```python
from build123d import *

# Parameters (mm, degrees)
F0_W     = 1.376042
F0_H     = 15
F1_DEPTH = 19
F2_R     = 5
F3_R     = 4.06
F4_DEPTH = 17
F5_R     = 4.15
F5_R_2   = 2.15
F6_DEPTH = 3


with BuildPart() as f1:
    # F0 (on Top) → F1 (new body)
    with BuildSketch(Plane.XY):
        with BuildLine():
            ThreePointArc((-27.724563, 11.37891), (-27.434191, 12.156994), (-27.831811, 12.886122))
            ThreePointArc((-27.831811, 12.886122), (-30.832093, 14.457622), (-34.175314, 15))
            Line((-34.175314, 15), (-34.175314, 12.15))
            ThreePointArc((-34.175314, 12.15), (-31.784278, 11.77065), (-29.628073, 10.669856))
            ThreePointArc((-29.628073, 10.669856), (-28.961501, 10.481293), (-28.332327, 10.771145))
            Line((-28.332327, 10.771145), (-27.724563, 11.37891))
        make_face()
        with BuildLine():
            Line((-34.175314, 12.15), (-34.175314, 15))
            ThreePointArc((-34.175314, 15), (-43.081071, 10.127467), (-43.78, 0))
            Line((-43.78, 0), (-40.507375, 0))
            ThreePointArc((-40.507375, 0), (-41.025816, 7.995189), (-34.175314, 12.15))
        make_face()
        with BuildLine():
            ThreePointArc((-43.78, 0), (-43.081071, 10.127467), (-34.175314, 15))
            Line((-34.175314, 15), (-50.774272, 15))
            Line((-50.774272, 15), (-50.774272, 0))
            Line((-50.774272, 0), (-43.78, 0))
        make_face()
        with BuildLine():
            Line((-40.507375, 0), (-43.78, 0))
            ThreePointArc((-43.78, 0), (-36.768247, -5.827186), (-27.829234, -4.03419))
            ThreePointArc((-27.829234, -4.03419), (-27.431848, -3.305092), (-27.72223, -2.52716))
            Line((-27.72223, -2.52716), (-28.329965, -1.919425))
            ThreePointArc((-28.329965, -1.919425), (-28.959306, -1.62956), (-29.625982, -1.818333))
            ThreePointArc((-29.625982, -1.818333), (-35.448544, -3.194351), (-40.507375, 0))
        make_face()
        with Locations((-51.462293, 7.5)):
            Rectangle(F0_W, F0_H)
        with BuildLine():
            Line((-52.150314, 15), (-50.774272, 15))
            Line((-50.774272, 15), (-50.774272, 16.6))
            ThreePointArc((-50.774272, 16.6), (-50.920718, 16.953553), (-51.274272, 17.1))
            Line((-51.274272, 17.1), (-52.150314, 17.1))
            Line((-52.150314, 17.1), (-52.150314, 15))
        make_face()
    extrude(amount=F1_DEPTH)

    # F2
    f2_edges = [f1.edges().sort_by_distance(p)[0] for p in [
        (-47.965157, 0, 19),
        (-47.965157, 0, 0),
    ]]
    fillet(f2_edges, radius=F2_R)

    # F3 (on face) → F4 (cut)
    with BuildSketch(Plane(origin=(-52.150314, 0, 0), x_dir=(0, -1, 0), z_dir=(-1, 0, 0))):
        with Locations((-8, 10)):
            Circle(F3_R)
    extrude(amount=-F4_DEPTH, mode=Mode.SUBTRACT)

    # F5 (on face) → F6 (join)
    with BuildSketch(Plane(origin=(-52.150314, 0, 0), x_dir=(0, -1, 0), z_dir=(-1, 0, 0))):
        with Locations((-8, 10)):
            Circle(F5_R)
        with Locations((-8, 10)):
            Circle(F5_R_2, mode=Mode.SUBTRACT)
    extrude(amount=-F6_DEPTH)


solid = f1.part
```
Could you check a few things on this model? Use its own coordinates, in mm. A direction names the side the tool comes from. Round coordinates to 2 decimals unless told otherwise and drop trailing zeros. Loops run counter-clockwise (first coordinate to the right, second up) from the corner with the lowest first, then second, coordinate; pieces in that order, holes last. Notation, with made-up numbers: (-37.5, 48) -> (-14.5, 48) arc R28 ccw to (-14.5, 82) -> close; hole circle Ø4 at (59.25, 14). An arc over 180 degrees is marked (long way). One line per question, with ' | ' between items.
(1) If we section it at C-C on x = -31.5: List the corners of the cut face in (y, z) for me.
Model answer:
outline: (-5.81, 0) -> (-2.82, 0) -> (-2.82, 19) -> (-5.81, 19) -> close; (11.67, 0) -> (14.66, 0) -> (14.66, 19) -> (11.67, 19) -> close
(2) If we section it at D-D on y = 8: List the corners of the cut face in (x, z) for me, and give its area (3 significant figures).
Model answer:
outline: (-52.15, 0) -> (-41.02, 0) -> (-41.02, 5.94) -> (-49.15, 5.94) -> (-49.15, 7.85) -> (-52.15, 7.85) -> close; (-52.15, 12.15) -> (-49.15, 12.15) -> (-49.15, 14.06) -> (-41.02, 14.06) -> (-41.02, 19) -> (-52.15, 19) -> close | area: 133 mm^2
(3) If I drill on probe 1 along Z at (x, y) = (-49.75, 8); probe 2 along Y at (x, z) = (-35.5, 8.75); probe 3 along Y at (x, z) = (-39.25, 10.75), over which ranges is the centre line in solid material (lowest first)?
Model answer:
probe 1: z = 0 to 7.85, 12.15 to 19 | probe 2: y = -6.07 to -3.19, 12.04 to 15 | probe 3: y = -4.85 to -1.4, 11.99 to 15
(4) For pin 1 Ø8.5 at (x, z) = (-39.5, 10.5) entering from +Y; pin 2 Ø4 at (y, z) = (10, 11) entering from +X; pin 3 Ø5 at (x, z) = (-44, 6) entering from -Y, each with a flat end and sliding along its axis, tell me the tip position at first contact or that it passes through.
Model answer:
pin 1: stops at y = 15 | pin 2: stops at x = -27.44 | pin 3: stops at y = -3.2
(5) Thinking about a two-plate mould opening in Y: for faces 4 (the face through (-30.787, 14.442, 9.367)), 5 (the face through (-28.97, 10.48, 9.37)), 6 (the face through (-43, 8, 19)), 7 (the face through (-48, 0, 9)), which applies, released by +Y, released by -Y, zero draft, split by the parting line, or undercut?
Model answer:
face 4: released by +Y | face 5: undercut | face 6: zero draft | face 7: released by -Y
(6) If we section it at B-B on z = 10: List the corners of the cut face in (x, y) for me (3 decimals), and give its area (3 significant figures).
Model answer:
outline: (-52.15, 0) -> (-43.78, 0) arc R10.575 ccw to (-27.829, -4.034) arc R1 ccw to (-27.722, -2.527) -> (-28.33, -1.919) arc R1 ccw to (-29.626, -1.818) arc R7.725 cw to (-41.885, 3.94) -> (-49.15, 3.94) -> (-49.15, 5.85) -> (-52.15, 5.85) -> close; (-52.15, 10.15) -> (-49.15, 10.15) -> (-49.15, 12.06) -> (-35.351, 12.06) arc R7.725 cw to (-29.628, 10.67) arc R1 ccw to (-28.332, 10.771) -> (-27.725, 11.379) arc R1 ccw to (-27.832, 12.886) arc R10.575 ccw to (-34.175, 15) -> (-50.774, 15) -> (-50.774, 16.6) arc R0.5 ccw to (-51.274, 17.1) -> (-52.15, 17.1) -> close | area: 175 mm^2
(7) For faces 1 (the face through (-48, 1, 2)), 2 (the face through (-49.15, 6, 8)), 3 (the face through (-42, 15, 9)), which set-ups out of +Z, -Z, +X, -X, +Y, -Y let a thin tool reach every point of the face, with its end or its side?
Model answer:
face 1: -Z, -X, -Y | face 2: none | face 3: +Z, -Z, +X, +Y
(8) If we section it at A-A on x = -49.5: List the corners of the cut face in (y, z) for me.
Model answer:
outline: (0, 5) arc R5 ccw to (5, 0) -> (15, 0) -> (15, 19) -> (5, 19) arc R5 ccw to (0, 14) -> close; hole circle Ø4.3 at (8, 10)
